Check sheet for the modelled part. Datum: model origin and axes. Units: mm. Face numbers are marked on the shaded views. A direction names the side the tool comes from. Round coordinates to 2 decimals unless told otherwise and drop trailing zeros. Write each loop counter-clockwise with the first axis right and the second up, starting at its lowest first coordinate (ties: lowest second). Pieces come first, ordered by that corner, then holes. Notation, with made-up numbers: M -15.75,86.25 L 7.25,86.25 A16 ccw 7.25,110.25 Z; hole C 0,-3 d10. An arc over 180 degrees is marked long. Answer in a Markdown table with one row per item.
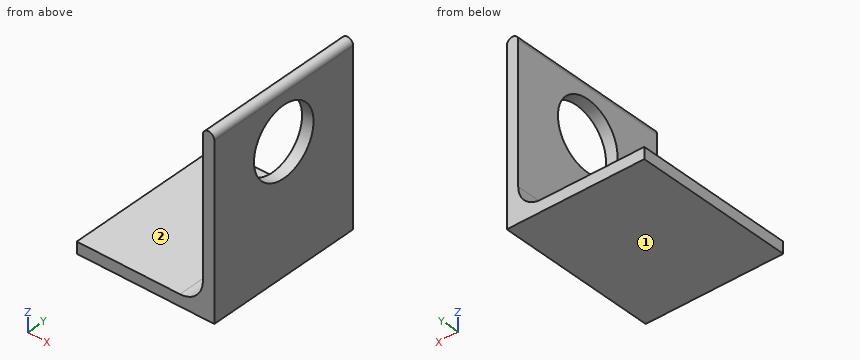
```python
from build123d import *

# Parameters (mm, degrees)
F1_DEPTH = 44.45
F3_D     = 19.05
F3_DEPTH = 25.4


with BuildPart() as f1:
    # F0 (on Front) → F1 (new body)
    with BuildSketch(Plane.XZ):
        with BuildLine():
            Line((28.575, 0), (0, 0))
            Line((0, 0), (0, -3.175))
            Line((0, -3.175), (34.925, -3.175))
            Line((34.925, -3.175), (38.1, -3.175))
            Line((38.1, -3.175), (38.1, 44.45))
            ThreePointArc((38.1, 44.45), (36.5125, 46.0375), (34.925, 44.45))
            Line((34.925, 44.45), (34.925, 6.35))
            ThreePointArc((34.925, 6.35), (33.065128, 1.859872), (28.575, 0))
        make_face()
    extrude(amount=F1_DEPTH)

    # F3
    with Locations(Plane.YZ.offset(38.1)):
        with Locations((-22.225, 31.828932)):
            Hole(F3_D / 2, depth=F3_DEPTH)


solid = f1.part
```
1. Section check C-C, the plane x = 36.5. Record the cut outline in (y, z) (3 decimals), and give its area (3 significant figures).
Found:
| item | result |
|---|---|
| outline | M -44.45,-3.175 L 0,-3.175 L 0,46.037 L -44.45,46.037 Z; hole C -22.225,31.829 d19.05 |
| area | 1,900 mm2 |
2. Go/stop test with flat-tipped pins: pin 1 (6 mm diameter, centred on x = 34, z = 10.5, fed in from -Y); pin 2 (8.5 mm diameter, centred on x = 20, y = -17, fed in from +Z); pin 3 (5 mm diameter, centred on y = -22.5, z = 4.5, fed in from -X); pin 4 (11.5 mm diameter, centred on y = -20, z = 23.5, fed in from -X) (3 decimals). Record where each tip stops, or that it passes through.
Found:
| item | result |
|---|---|
| pin 1 | stops at y = -44.45 |
| pin 2 | stops at z = 0 |
| pin 3 | stops at x = 33.2 |
| pin 4 | stops at x = 34.925 |
3. Access from +Z, -Z, +X, -X, +Y, -Y to the whole of each face (thin tool, end or side, straight path). Record for the marked faces 1 and 2.
Found:
| item | result |
|---|---|
| face 1 | -Z, +X, -X, +Y, -Y |
| face 2 | +Z, -X, +Y, -Y |
4. Section check D-D, the plane x = 27. Record the cut outline in (y, z) (3 decimals).
Found:
| item | result |
|---|---|
| outline | M -44.45,-3.175 L 0,-3.175 L 0,0 L -44.45,0 Z |
5. Scan lines: L1, parallel to Z at x = 23, y = -7 (3 decimals); L2, parallel to X at y = -30.5, z = 41 (3 decimals); L3, parallel to Z at x = 32.5, y = -41.5 (3 decimals). Record each from-to range of solid material in increasing order.
Found:
| item | result |
|---|---|
| L1 | z = -3.175 to 0 |
| L2 | x = 34.925 to 38.1 |
| L3 | z = -3.175 to 1.358 |
